from build123d import *

# Parameters (mm, degrees)
SKETCH1_R      = 1.395
EXTRUDE1_DEPTH = 4.955
EXTRUDE2_DEPTH = 3.105
EXTRUDE3_DEPTH = 2.415
EXTRUDE4_DEPTH = 2.92
EXTRUDE5_REACH = 16.985
SKETCH5_W      = 6.985
SKETCH5_H      = 0.53875
SKETCH5_R      = 0.6985
SKETCH6_R      = 0.635
EXTRUDE7_DEPTH = 1.508
SKETCH_R       = 1.395
EXTRUDE8_DEPTH = 7.92
FILLET1_R      = 1


with BuildPart() as part:
    # Sketch1 → Extrude1 (new body, symmetric)
    with BuildSketch(Plane.XY):
        with Locations((-11.3, 5.08)):
            Circle(SKETCH1_R)
        with BuildLine():
            Line((13.97, -5.334), (13.97, 5.334))
            ThreePointArc((13.97, 5.334), (13.226051224, 7.130051224), (11.43, 7.874))
            Line((11.43, 7.874), (-11.43, 7.874))
            ThreePointArc((-11.43, 7.874), (-13.226051224, 7.130051224), (-13.97, 5.334))
            Line((-13.97, 5.334), (-13.97, 3.048))
            Line((-13.97, 3.048), (-14.732, 3.048))
            Line((-14.732, 3.048), (-14.732, -4.572))
            Line((-14.732, -4.572), (-13.97, -4.572))
            Line((-13.97, -4.572), (-13.97, -5.334))
            ThreePointArc((-13.97, -5.334), (-13.226051224, -7.130051224), (-11.43, -7.874))
            Line((-11.43, -7.874), (11.43, -7.874))
            ThreePointArc((11.43, -7.874), (13.226051224, -7.130051224), (13.97, -5.334))
        make_face()
        with Locations((11.3, -5.16)):
            Circle(SKETCH1_R, mode=Mode.SUBTRACT)
        with Locations((-11.3, 5.08)):
            Circle(SKETCH1_R, mode=Mode.SUBTRACT)
        with Locations((11.3, -5.16)):
            Circle(SKETCH1_R)
    extrude(amount=EXTRUDE1_DEPTH, both=True)

    # Sketch2 → Extrude2 (add, symmetric)
    with BuildSketch(Plane.XY):
        Polygon((-17.907, -2.286), (-17.907, -10.795), (-17.399, -10.795), (-17.399, -2.794), (-14.732, -2.794), (-14.732, -2.286), align=None)
    extrude(amount=EXTRUDE2_DEPTH, both=True)

    # Sketch3 → Extrude3 (add, symmetric)
    with BuildSketch(Plane.XY):
        with BuildLine():
            Line((10.16, 7.874), (10.16, 9.139))
            ThreePointArc((10.16, 9.139), (8.89, 10.409), (7.62, 9.139))
            Line((7.62, 9.139), (7.62, 7.874))
            Line((7.62, 7.874), (10.16, 7.874))
        make_face()
    extrude(amount=EXTRUDE3_DEPTH, both=True)

    # Sketch4 → Extrude4 (add, symmetric)
    with BuildSketch(Plane.XY):
        Polygon((-0.38, -18.034), (-0.38, -10.984), (-1.015, -11.05270614), (-1.015, -18.034), align=None)
        Polygon((-1.015, -11.05270614), (-0.38, -10.984), (-0.38, -7.874), (-1.015, -7.874), (-1.015, -10.414), align=None)
    extrude(amount=EXTRUDE4_DEPTH, both=True)

    # Sketch5 → Extrude5 (cut, up to next)
    with BuildSketch(Plane(origin=(-1.015, -13.250765139, 0), x_dir=(0, -1, 0), z_dir=(-1, 0, 0)), mode=Mode.PRIVATE) as extrude5_sk1:
        with Locations((1.290734861, -2.650625)):
            Rectangle(SKETCH5_W, SKETCH5_H)
    extrude5_tool1 = extrude(extrude5_sk1.sketch, amount=-EXTRUDE5_REACH, mode=Mode.PRIVATE) & part.part
    add(extrude5_tool1.solids().sort_by_distance((-1.015, -14.5415, -2.650625))[0], mode=Mode.SUBTRACT)
    # Sketch5 → Extrude5 (cut, up to next)
    with BuildSketch(Plane(origin=(-1.015, -13.250765139, 0), x_dir=(0, -1, 0), z_dir=(-1, 0, 0)), mode=Mode.PRIVATE) as extrude5_sk2:
        with Locations((1.290734861, 2.650625)):
            Rectangle(SKETCH5_W, SKETCH5_H)
    extrude5_tool2 = extrude(extrude5_sk2.sketch, amount=-EXTRUDE5_REACH, mode=Mode.PRIVATE) & part.part
    add(extrude5_tool2.solids().sort_by_distance((-1.015, -14.5415, 2.650625))[0], mode=Mode.SUBTRACT)
    # Sketch5 → Extrude5 (cut, up to next)
    with BuildSketch(Plane(origin=(-1.015, -13.250765139, 0), x_dir=(0, -1, 0), z_dir=(-1, 0, 0)), mode=Mode.PRIVATE) as extrude5_sk3:
        with Locations((1.608234861, 0)):
            Circle(SKETCH5_R)
    extrude5_tool3 = extrude(extrude5_sk3.sketch, amount=-EXTRUDE5_REACH, mode=Mode.PRIVATE) & part.part
    add(extrude5_tool3.solids().sort_by_distance((-1.015, -14.859, 0))[0], mode=Mode.SUBTRACT)

    # Sketch6 → Extrude7 (cut, through all)
    with BuildSketch(Plane(origin=(-17.399, 14.605, 0), x_dir=(0, 1, 0), z_dir=(1, 0, 0))):
        with Locations((-22.352, 0)):
            Circle(SKETCH6_R)
    extrude(amount=-EXTRUDE7_DEPTH, mode=Mode.SUBTRACT)

    # Sketch → Extrude8 (cut, symmetric)
    with BuildSketch(Plane.XY):
        with Locations((-11.3, 5.08)):
            Circle(SKETCH_R)
        with Locations((11.3, -5.16)):
            Circle(SKETCH_R)
    extrude(amount=EXTRUDE8_DEPTH, both=True, mode=Mode.SUBTRACT)

    # Fillet1
    fillet1_edges = [part.edges().sort_by_distance(p)[0] for p in [
        (-17.907, -2.286, 0),
        (-17.399, -2.794, 0),
    ]]
    fillet(fillet1_edges, radius=FILLET1_R)


solid = part.part
Model file for the job. Use its own axes, mm. A direction names the side the tool comes from. Round coordinates to 2 decimals unless told otherwise and drop trailing zeros. Order: outer loops, then holes, each group sorted by start corner. A loop starts at its lowest first (then second) coordinate and runs counter-clockwise, first axis right, second up.
(1) Band-saw the part on C-C (x = -12). List the corners of the cut face in (y, z) (3 decimals), then the cut area to 3 significant figures.
(2) Drill centre lines: line 1 (Y direction, x = -11.3, z = -0.25) (3 decimals); line 2 (Y direction, x = 11.3, z = 2.25) (3 decimals); line 3 (Y direction, x = -7, z = -1.5). Where is each one in solid material? Low to high.
(3) Band-saw the part on B-B (x = 8.89). List the corners of the cut face in (y, z) (3 decimals).
(4) Pin check, flat tips, straight feed: pin 1 (1 mm diameter, centred on y = 3.5, z = -2.5, fed in from -X); pin 2 (5 mm diameter, centred on x = 4.5, z = -1, fed in from -Y); pin 3 (0.6 mm diameter, centred on y = 8.5, z = 0.5, fed in from -X); pin 4 (1.7 mm diameter, centred on x = 11.3, y = -5.16, fed in from -Z). Stop position of each tip, or through.
(5) Band-saw the part on D-D (y = -15). List the corners of the cut face in (x, z) (3 decimals), then the cut area to 3 significant figures.
(6) Pull direction X, two halves, no side cores. Call faces 1 (the face through (13.246, 7.11, 0.069)), 2 (the face through (-12.407, 4.231, -0.069)), 3 (the face through (7.62, 8.5, 0)): released by +X, released by -X, zero draft, split by the parting line, or undercut.
(7) 3-axis set-ups, long thin cutter, end or side, ignore diameter. For faces 4 (the face through (-1.015, -13, 0)), 5 (the face through (9, 9, 2.415)), 6 (the face through (-0.38, -13, 0)), 7 (the face through (-13.97, 4, 0)): which of +Z, -Z, +X, -X, +Y, -Y reach the whole face in a straight line?
(8) Band-saw the part on A-A (z = -3.75). List the corners of the cut face in (x, y) (3 decimals), then the cut area to 3 significant figures.
Verdict:
1. outline: (-7.809, -4.955) - (3.873, -4.955) - (3.873, 4.955) - (-7.809, 4.955) - close; (6.287, -4.955) - (7.809, -4.955) - (7.809, 4.955) - (6.287, 4.955) - close
1. area: 131 mm2
2. line 1: y = -7.874 to 3.685, 6.475 to 7.874
2. line 2: y = -7.874 to -6.555, -3.765 to 7.874
2. line 3: y = -7.87 to 7.87
3. outline: (-7.874, -4.955) - (7.874, -4.955) - (7.874, -2.415) - (10.409, -2.415) - (10.409, 2.415) - (7.874, 2.415) - (7.874, 4.955) - (-7.874, 4.955) - close
4. pin 1: stops at x = -14.73
4. pin 2: stops at y = -7.87
4. pin 3: stops at x = 7.62
4. pin 4: passes through
5. outline: (-1.015, -2.381) - (-0.38, -2.381) - (-0.38, -0.684) - (-1.015, -0.684) - close; (-1.015, 0.684) - (-0.38, 0.684) - (-0.38, 2.381) - (-1.015, 2.381) - close
5. area: 2.16 mm2
6. face 1: released by +X
6. face 2: undercut
6. face 3: released by -X
7. face 4: +Z, -Z, -Y
7. face 5: +Z, +X, -X, +Y
7. face 6: +Z, -Z, +X, -Y
7. face 7: +Z, -Z, -X, +Y
8. outline: (-14.732, -4.572) - (-13.97, -4.572) - (-13.97, -5.334) arc R2.54 ccw to (-11.43, -7.874) - (11.43, -7.874) arc R2.54 ccw to (13.97, -5.334) - (13.97, 5.334) arc R2.54 ccw to (11.43, 7.874) - (-11.43, 7.874) arc R2.54 ccw to (-13.97, 5.334) - (-13.97, 3.048) - (-14.732, 3.048) - close; hole circle Ø2.79 at (-11.3, 5.08); hole circle Ø2.79 at (11.3, -5.16)
8. area: 428 mm2
